Geometry: final body of the model. Coordinates: model frame, mm. A direction names the side the tool comes from. Give positions to 0.01 mm unless a question says otherwise; leave off trailing zeros. Write each loop counter-clockwise with the first axis right and the second up, starting at its lowest first coordinate (ties: lowest second). Pieces come first, ordered by that corner, then holes.
Q1. Reachability of faces 4 (the flat face through (0, 0, 28)), 5 (the flat face through (0, 9, 16)), 6 (the cylindrical face through (0.104, -2.126, 1.207)) from +Z, -Z, +X, -X, +Y, -Y: full face, straight path, thin tool, end or side. Return the list, or none.
Q2. Pin query (flat end, axial travel): pin 1 Ø1 at (y, z) = (8, 6) entering from +X; pin 2 Ø2.5 at (x, z) = (0.5, 4.5) entering from +Y; pin 3 Ø1.2 at (x, y) = (1, 8) entering from -Z; pin 4 Ø8 at (x, y) = (0, 0) entering from -Z. Return the tip coordinate at first contact, or that it passes through.
Q3. Line query: line 1 (Z direction, x = 0, y = -6.25); line 2 (Z direction, x = 0, y = 0.75); line 3 (Z direction, x = -1, y = 2.25). Output: solid intervals per line, ascending.
Q4. Section A-A (y = 0). Return the cut outline in (x, z), plus the area to 3 significant figures.
Q5. Section D-D (x = 6.5). Return the cut outline in (y, z).
Q6. Section C-C (z = 28.5). Return the cut outline in (x, y).
Q7. Mould query, pull axis Y, two halves, no side actions, for faces 1 (the flat face through (0, 7, 8)), 2 (the flat face through (4, 9, 8)), 3 (the cylindrical face through (-0.54, -2.44, 32.06)). Classes: +Y half, -Y half, draft (parallel to the pull), parting line (faces both ways), or undercut.
Q8. Section B-B (z = 2). Return the cut outline in (x, y).
from build123d import *

# Parameters (mm, degrees)
SKETCH1_R             = 11
BOSS_EXTRUDE1_DEPTH   = 36
SKETCH2_W             = 8
SKETCH2_H             = 30
CUT_EXTRUDE1_DEPTH    = 16
CUT_EXTRUDE3_START    = -10
CUT_EXTRUDE3_DEPTH    = 10
M2X0_4_TAPPED_HOLE3_D = 1.6
SKETCH16_R            = 2.5
CUT_EXTRUDE4_DEPTH    = 8


with BuildPart() as part:
    # Sketch1 → Boss-Extrude1 (new body)
    with BuildSketch(Plane.XY):
        Circle(SKETCH1_R)
    extrude(amount=BOSS_EXTRUDE1_DEPTH)

    # Sketch2 → Cut-Extrude1 (cut)
    with BuildSketch(Plane(origin=(0, 0, 0), x_dir=(-1, 0, 0), z_dir=(0, 0, -1))):
        with Locations((0, 22)):
            Rectangle(SKETCH2_W, SKETCH2_H)
    extrude(amount=-CUT_EXTRUDE1_DEPTH, mode=Mode.SUBTRACT)

    # Sketch6 → Cut-Extrude3 (cut)
    with BuildSketch(Plane.XY.offset(36).offset(CUT_EXTRUDE3_START)):
        with BuildLine():
            Line((-0.286520362, 10.996267825), (0, 10.5))
            Line((0, 10.5), (0.286520362, 10.996267825))
            ThreePointArc((0.286520362, 10.996267825), (0, 11), (-0.286520362, 10.996267825))
        make_face()
    extrude(amount=CUT_EXTRUDE3_DEPTH, mode=Mode.SUBTRACT)

    # M2x0.4 Tapped Hole3 (through all)
    with Locations(Plane(origin=(0, 7, 0), x_dir=(1, 0, 0), z_dir=(0, 1, 0))):
        with Locations((0, -12), (0, -2)):
            Hole(M2X0_4_TAPPED_HOLE3_D / 2)

    # Sketch16 → Cut-Extrude4 (cut)
    with BuildSketch(Plane.XY.offset(36)):
        Circle(SKETCH16_R)
    extrude(amount=-CUT_EXTRUDE4_DEPTH, mode=Mode.SUBTRACT)


solid = part.part
Computed:
1. face 4: +Z
1. face 5: -Z, +Y
1. face 6: +Y, -Y
2. pin 1: stops at x = 8.05
2. pin 2: stops at y = 7
2. pin 3: stops at z = 16
2. pin 4: stops at z = 0
3. line 1: z = 0 to 1.2, 2.8 to 11.2, 12.8 to 36
3. line 2: z = 0 to 1.2, 2.8 to 11.2, 12.8 to 28
3. line 3: z = 0 to 28
4. outline: (-11, 0) - (11, 0) - (11, 36) - (2.5, 36) - (2.5, 28) - (-2.5, 28) - (-2.5, 36) - (-11, 36) - close; hole circle Ø1.6 at (0, 2); hole circle Ø1.6 at (0, 12)
4. area: 748 mm2
5. outline: (-8.87, 0) - (8.87, 0) - (8.87, 36) - (-8.87, 36) - close
6. outline: (-0.29, 11) arc R11 ccw (long way) to (0.29, 11) - (0, 10.5) - close; hole circle Ø5 at (0, 0)
7. face 1: +Y half
7. face 2: draft
7. face 3: undercut
8. outline: (-4, 7) - (-4, 10.25) arc R11 ccw to (-0.8, -10.97) - (-0.8, 7) - close; (0.8, -10.97) arc R11 ccw to (4, 10.25) - (4, 7) - (0.8, 7) - close
